Work out the finished part from the listing and answer in its coordinate system (mm). Round coordinates to 2 decimals unless told otherwise and drop trailing zeros. Write each loop counter-clockwise with the first axis right and the second up, starting at its lowest first coordinate (ties: lowest second). Pieces come first, ordered by that corner, then holes. Notation, with made-up numbers: M 34.5,32 L 45.5,32 A20 ccw 45.5,54 Z; hole C -31,-22 d10. An arc over 180 degrees is marked long. One line per item, written item: value. Start each with the question number.
Q1. Given pin 1 Ø3.5 at (y, z) = (3.5, 4.5) entering from +X; pin 2 Ø3 at (x, y) = (19.5, 3) entering from -Z; pin 3 Ø3 at (x, y) = (116, 4) entering from +Z, each flat-ended and moving along its own axis, determine where each tip first touches the part or whether it passes through.
Q2. Find section C-C (y = 2.55). Count the separate pieces of the cut face and the enclosed holes in it, and give its area (3 significant figures).
Q3. Consider probe 1 along X at (y, z) = (2.15, 41.5); probe 2 along X at (y, z) = (4.85, 25); probe 3 along X at (y, z) = (5.85, 29). Determine where each line is inside the solid, lowest interval first.
Q4. Find section B-B (z = 8.5). Write down the section's boundary in (x, y).
Q5. Find section A-A (x = 79). Write down the section's boundary in (y, z), and give its area (3 significant figures).
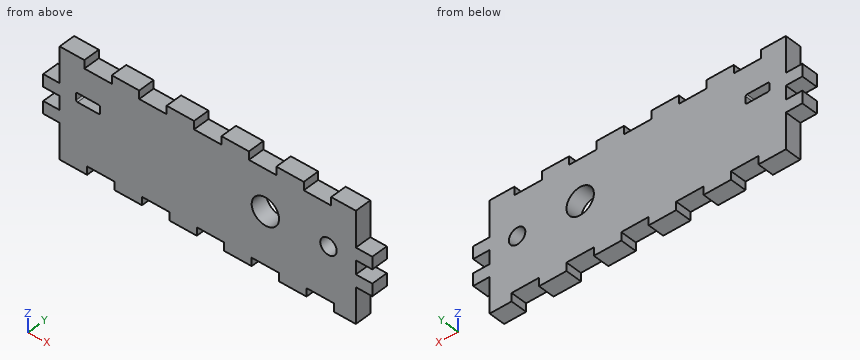
from build123d import *

# Parameters (mm, degrees)
SKETCH_1_W          = 112
SKETCH_1_H          = 40
EXTRUDE_1_DEPTH     = 6
SKETCH_2_R          = 3
CUT_EXTRUDE_1_DEPTH = 120.079805173
CUT_EXTRUDE_2_DEPTH = 10
SKETCH_4_R          = 4.9895
CUT_EXTRUDE_3_DEPTH = 120.079805173
SKETCH_6_W          = 4.5
SKETCH_6_H          = 6
EXTRUDE_3_DEPTH     = 6
SKETCH_11_W         = 40
SKETCH_11_H         = 6
CUT_EXTRUDE_4_DEPTH = 4
SKETCH_12_W         = 4.5
SKETCH_12_H         = 6
EXTRUDE_10_DEPTH    = 6
SKETCH_13_W         = 9
SKETCH_13_H         = 6
SKETCH_13_W_2       = 10
EXTRUDE_11_DEPTH    = 3
SKETCH_14_W         = 108
SKETCH_14_H         = 6
CUT_EXTRUDE_5_DEPTH = 2
SKETCH_15_W         = 108
SKETCH_15_H         = 6
CUT_EXTRUDE_6_DEPTH = 2
SKETCH_16_W         = 10
SKETCH_16_H         = 6
CUT_EXTRUDE_7_DEPTH = 3
SKETCH_17_W         = 10
SKETCH_17_H         = 6
SKETCH_17_W_2       = 8
EXTRUDE_12_DEPTH    = 1
SKETCH_18_W         = 10
SKETCH_18_H         = 6
EXTRUDE_13_DEPTH    = 1


with BuildPart() as part:
    # Эскиз1 → Бобышка-Вытянуть1 (new body)
    with BuildSketch(Plane(origin=(0, 0, 0), x_dir=(1, 0, 0), z_dir=(0, 1, 0))):
        with Locations((56, -20)):
            Rectangle(SKETCH_1_W, SKETCH_1_H)
    extrude(amount=EXTRUDE_1_DEPTH)

    # Эскиз2 → Вырез-Вытянуть1 (cut, through all)
    with BuildSketch(Plane(origin=(0, 6, 0), x_dir=(1, 0, 0), z_dir=(0, 1, 0))):
        with Locations(Location((102, -25, 0), (0, 0, 270))):
            Circle(SKETCH_2_R)
    extrude(amount=-CUT_EXTRUDE_1_DEPTH, mode=Mode.SUBTRACT)

    # Эскиз3 → Вырез-Вытянуть2 (cut)
    with BuildSketch(Plane(origin=(0, 6, 0), x_dir=(1, 0, 0), z_dir=(0, 1, 0))):
        with BuildLine():
            Line((10.5, -26.78), (18.17, -26.78))
            ThreePointArc((18.17, -26.78), (18.523553391, -26.926446609), (18.67, -27.28))
            Line((18.67, -27.28), (18.67, -29.5))
            ThreePointArc((18.67, -29.5), (18.523553391, -29.853553391), (18.17, -30))
            Line((18.17, -30), (10.5, -30))
            ThreePointArc((10.5, -30), (10.146446609, -29.853553391), (10, -29.5))
            Line((10, -29.5), (10, -27.28))
            ThreePointArc((10, -27.28), (10.146446609, -26.926446609), (10.5, -26.78))
        make_face()
    extrude(amount=-CUT_EXTRUDE_2_DEPTH, mode=Mode.SUBTRACT)

    # Эскиз4 → Вырез-Вытянуть3 (cut, through all)
    with BuildSketch(Plane(origin=(0, 6, 0), x_dir=(1, 0, 0), z_dir=(0, 1, 0))):
        with Locations(Location((79, -25, 0), (0, 0, 270))):
            Circle(SKETCH_4_R)
    extrude(amount=-CUT_EXTRUDE_3_DEPTH, mode=Mode.SUBTRACT)

    # Эскиз6 → Бобышка-Вытянуть3 (add)
    with BuildSketch(Plane(origin=(112, 0, 0), x_dir=(0, 0, -1), z_dir=(1, 0, 0))):
        with Locations((-27.75, 3)):
            Rectangle(SKETCH_6_W, SKETCH_6_H)
        with Locations((-18.25, 3)):
            Rectangle(SKETCH_6_W, SKETCH_6_H)
    extrude(amount=EXTRUDE_3_DEPTH)

    # Эскиз11 → Вырез-Вытянуть4 (cut)
    with BuildSketch(Plane.ZY):
        with Locations((20, 3)):
            Rectangle(SKETCH_11_W, SKETCH_11_H)
    extrude(amount=-CUT_EXTRUDE_4_DEPTH, mode=Mode.SUBTRACT)

    # Эскиз12 → Бобышка-Вытянуть10 (add)
    with BuildSketch(Plane.ZY.offset(-4)):
        with Locations((18.25, 3)):
            Rectangle(SKETCH_12_W, SKETCH_12_H)
        with Locations((27.75, 3)):
            Rectangle(SKETCH_12_W, SKETCH_12_H)
    extrude(amount=EXTRUDE_10_DEPTH)

    # Эскиз13 → Бобышка-Вытянуть11 (add)
    with BuildSketch(Plane.XY.offset(40)):
        with Locations((8.5, 3)):
            Rectangle(SKETCH_13_W, SKETCH_13_H)
        with Locations((107.5, 3)):
            Rectangle(SKETCH_13_W, SKETCH_13_H)
        with Locations((28, 3)):
            Rectangle(SKETCH_13_W_2, SKETCH_13_H)
        with Locations((48, 3)):
            Rectangle(SKETCH_13_W_2, SKETCH_13_H)
        with Locations((68, 3)):
            Rectangle(SKETCH_13_W_2, SKETCH_13_H)
        with Locations((88, 3)):
            Rectangle(SKETCH_13_W_2, SKETCH_13_H)
    extrude(amount=EXTRUDE_11_DEPTH)

    # Эскиз14 → Вырез-Вытянуть5 (cut)
    with BuildSketch(Plane(origin=(0, 0, 0), x_dir=(-1, 0, 0), z_dir=(0, 0, -1))):
        with Locations((-58, 3)):
            Rectangle(SKETCH_14_W, SKETCH_14_H)
    extrude(amount=-CUT_EXTRUDE_5_DEPTH, mode=Mode.SUBTRACT)

    # Эскиз15 → Вырез-Вытянуть6 (cut)
    with BuildSketch(Plane(origin=(0, 0, 2), x_dir=(-1, 0, 0), z_dir=(0, 0, -1))):
        with Locations((-58, 3)):
            Rectangle(SKETCH_15_W, SKETCH_15_H)
    extrude(amount=-CUT_EXTRUDE_6_DEPTH, mode=Mode.SUBTRACT)

    # Эскиз16 → Вырез-Вытянуть7 (cut)
    with BuildSketch(Plane(origin=(0, 0, 4), x_dir=(-1, 0, 0), z_dir=(0, 0, -1))):
        with Locations((-19, 3)):
            Rectangle(SKETCH_16_W, SKETCH_16_H)
        with Locations((-39, 3)):
            Rectangle(SKETCH_16_W, SKETCH_16_H)
        with Locations((-59, 3)):
            Rectangle(SKETCH_16_W, SKETCH_16_H)
        with Locations((-79, 3)):
            Rectangle(SKETCH_16_W, SKETCH_16_H)
        with Locations((-99, 3)):
            Rectangle(SKETCH_16_W, SKETCH_16_H)
    extrude(amount=-CUT_EXTRUDE_7_DEPTH, mode=Mode.SUBTRACT)

    # Эскиз17 → Бобышка-Вытянуть12 (add)
    with BuildSketch(Plane(origin=(0, 0, 4), x_dir=(-1, 0, 0), z_dir=(0, 0, -1))):
        with Locations((-9, 3)):
            Rectangle(SKETCH_17_W, SKETCH_17_H)
        with Locations((-29, 3)):
            Rectangle(SKETCH_17_W, SKETCH_17_H)
        with Locations((-49, 3)):
            Rectangle(SKETCH_17_W, SKETCH_17_H)
        with Locations((-69, 3)):
            Rectangle(SKETCH_17_W, SKETCH_17_H)
        with Locations((-89, 3)):
            Rectangle(SKETCH_17_W, SKETCH_17_H)
        with Locations((-108, 3)):
            Rectangle(SKETCH_17_W_2, SKETCH_17_H)
    extrude(amount=EXTRUDE_12_DEPTH)

    # Эскиз18 → Бобышка-Вытянуть13 (add)
    with BuildSketch(Plane(origin=(0, 0, 7), x_dir=(-1, 0, 0), z_dir=(0, 0, -1))):
        with Locations((-19, 3)):
            Rectangle(SKETCH_18_W, SKETCH_18_H)
        with Locations((-39, 3)):
            Rectangle(SKETCH_18_W, SKETCH_18_H)
        with Locations((-59, 3)):
            Rectangle(SKETCH_18_W, SKETCH_18_H)
        with Locations((-79, 3)):
            Rectangle(SKETCH_18_W, SKETCH_18_H)
        with Locations((-99, 3)):
            Rectangle(SKETCH_18_W, SKETCH_18_H)
    extrude(amount=EXTRUDE_13_DEPTH)


solid = part.part
The answers:
1. pin 1: x = 112
1. pin 2: z = 6
1. pin 3: z = 30
2. separate pieces: 1
2. enclosed holes: 3
2. area: 3,990 mm2
3. probe 1: 4 to 13, 23 to 33, 43 to 53, 63 to 73, 83 to 93, 103 to 112
3. probe 2: 4 to 74.01, 83.99 to 99, 105 to 112
3. probe 3: -2 to 10, 18.67 to 76.02, 81.98 to 118
4. outline: M 4,0 L 112,0 L 112,6 L 4,6 Z
5. outline: M 0,6 L 6,6 L 6,20.01 L 0,20.01 Z; M 0,29.99 L 6,29.99 L 6,40 L 0,40 Z
5. area: 144 mm2
